Could you check a few things on this drawing? It's one solid part, dimensions in mm from its lowest x, y, z. Give positions to 0.01 mm unless a question says otherwise; leave off trailing zeros. Order: outer loops, then holes, each group sorted by start corner. A loop starts at its lowest first (then second) coordinate and runs counter-clockwise, first axis right, second up. Notation, with made-up numbers: (-1, 9.5) - (23, 9.5) arc R10 ccw to (23, 15.5) - close; hole circle Ø6 at (80.5, 31.5). An arc over 180 degrees is marked (long way). Put each result on its own line as item: value.
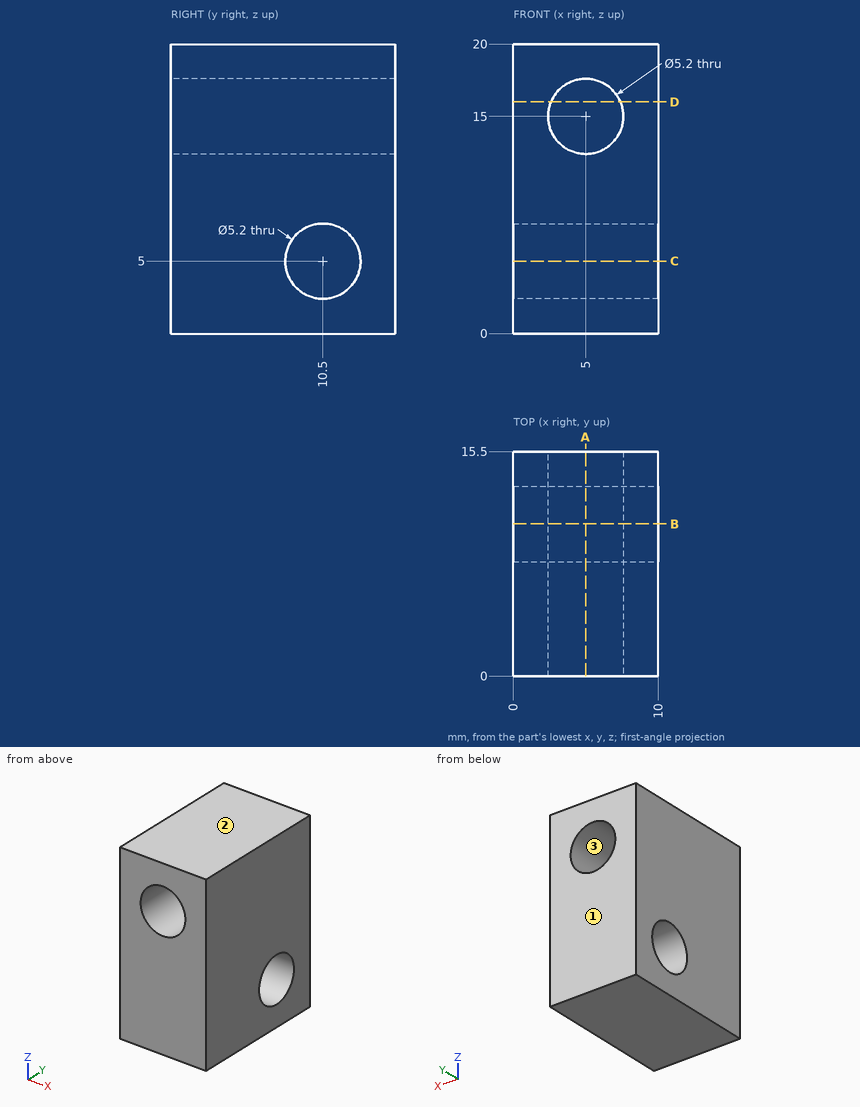
1) We'd pull the mould along Z, two halves only. Please class the marked faces 1, 2 and 3: pulls with the +Z half, pulls with the -Z half, needs draft (parallel to the pull), parting line crosses it, or undercut.
Filled in:
face 1: needs draft
face 2: pulls with the +Z half
face 3: undercut
2) If I drill on line 1 (Z direction, x = 5, y = 6.5); line 2 (Z direction, x = 6.75, y = 8.5); line 3 (Z direction, x = 5, y = 11), over which ranges is the centre line in solid material (lowest first)? Write a range as [from, to].
Filled in:
line 1: z = [0, 12.4], [17.6, 20]
line 2: z = [0, 3.34], [6.66, 13.08], [16.92, 20]
line 3: z = [0, 2.45], [7.55, 12.4], [17.6, 20]
3) Suppose I cut it at B-B, the plane y = 10.5. List the corners of the cut face in (x, z) for me, and give its area (3 significant figures).
Filled in:
outline: (0, 0) - (10, 0) - (10, 2.4) - (0, 2.4) - close; (0, 7.6) - (10, 7.6) - (10, 20) - (0, 20) - close; hole circle Ø5.2 at (5, 15)
area: 127 mm^2
4) I'm going to push a flat-ended pin straight in: pin 1 (4.5 mm diameter, centred on x = 5, z = 15, fed in from +Y). Where does the tip first touch, or does it pass through?
Filled in:
pin 1: passes through
5) Suppose I cut it at D-D, the plane z = 16. List the corners of the cut face in (x, y) for me.
Filled in:
outline: (0, 0) - (2.6, 0) - (2.6, 15.5) - (0, 15.5) - close; (7.4, 0) - (10, 0) - (10, 15.5) - (7.4, 15.5) - close
6) Suppose I cut it at C-C, the plane z = 5. List the corners of the cut face in (x, y) for me.
Filled in:
outline: (0, 0) - (10, 0) - (10, 7.9) - (0, 7.9) - close; (0, 13.1) - (10, 13.1) - (10, 15.5) - (0, 15.5) - close
7) Suppose I cut it at A-A, the plane x = 5. List the corners of the cut face in (y, z) for me, and give its area (3 significant figures).
Filled in:
outline: (0, 0) - (15.5, 0) - (15.5, 12.4) - (0, 12.4) - close; (0, 17.6) - (15.5, 17.6) - (15.5, 20) - (0, 20) - close; hole circle Ø5.2 at (10.5, 5)
area: 208 mm^2
